from build123d import *

# Parameters (mm, degrees)
SKETCH1_W           = 44
SKETCH1_H           = 30
BOSS_EXTRUDE1_DEPTH = 3
SKETCH2_R           = 1
CUT_EXTRUDE1_DEPTH  = 5
SKETCH3_R           = 1
CUT_EXTRUDE2_DEPTH  = 5


with BuildPart() as part:
    # Sketch1 → Boss-Extrude1 (new body)
    with BuildSketch(Plane(origin=(0, 0, 0), x_dir=(1, 0, 0), z_dir=(0, 1, 0))):
        Rectangle(SKETCH1_W, SKETCH1_H)
    extrude(amount=BOSS_EXTRUDE1_DEPTH)

    # Sketch2 → Cut-Extrude1 (cut)
    with BuildSketch(Plane.ZY.offset(22)):
        with Locations((0, 1.5)):
            Circle(SKETCH2_R)
    cut_extrude1 = extrude(amount=-CUT_EXTRUDE1_DEPTH, mode=Mode.SUBTRACT)

    # Mirror1: Cut-Extrude1 across plane
    add(cut_extrude1.mirror(Plane(origin=(0, 0, 0), x_dir=(0, 0, 1), z_dir=(1, 0, 0))), mode=Mode.SUBTRACT)

    # Sketch3 → Cut-Extrude2 (cut)
    with BuildSketch(Plane(origin=(0, 0, 0), x_dir=(-1, 0, 0), z_dir=(0, -1, 0))):
        with Locations(Location((15, 4.5, 0), (0, 0, 90))):
            Circle(SKETCH3_R)
        with Locations(Location((15, -12.5, 0), (0, 0, 90))):
            Circle(SKETCH3_R)
        with Locations(Location((-15, -12.5, 0), (0, 0, 90))):
            Circle(SKETCH3_R)
        with Locations(Location((-15, 4.5, 0), (0, 0, 90))):
            Circle(SKETCH3_R)
    extrude(amount=-CUT_EXTRUDE2_DEPTH, mode=Mode.SUBTRACT)


solid = part.part
Read the model definition and answer for the solid it produces. Units are mm, in the model's axes. A direction names the side the tool comes from. Give positions to 0.01 mm unless a question says otherwise; leave off trailing zeros. Write each loop counter-clockwise with the first axis right and the second up, starting at its lowest first coordinate (ties: lowest second). Pieces come first, ordered by that corner, then holes. Notation, with made-up numbers: (62.25, -32.75) -> (88.25, -32.75) arc R15 ccw to (88.25, -8.75) -> close; hole circle Ø10 at (-34, 88.5). An arc over 180 degrees is marked (long way). Answer as a JSON object with one key per item and string values. Group by question number.
1) Find section C-C (y = 0.95). Write down the section's boundary in (x, z), and give its area (3 significant figures).
2) This flat-tipped pin is pushed along its axis until it touches: P1, Ø1.6, axis at y = 1.5, z = 0, coming from the +X side. Where does it stop, or does it pass through?
3) Find section B-B (x = 15). Write down the section's boundary in (y, z), and give its area (3 significant figures).
4) Find section A-A (z = 12.5). Write down the section's boundary in (x, y), and give its area (3 significant figures).
5) Consider L1, parallel to X at y = 1.2, z = 12.5; L2, parallel to Y at x = -21, z = 0; L3, parallel to X at y = 0.65, z = 13.25. Determine where each line is inside the solid, lowest interval first. Write a range as from..to.
6) A tool of negligible diameter and unlimited length cuts with its end or side. For faces 4 (the cylindrical face through (19.535, 0.524, -0.217)), 5 (the flat face through (22, 2.8, 0.2)), 6 (the cylindrical face through (-19.535, 0.524, -0.217)), from which of +Z, -Z, +X, -X, +Y, -Y can it reach the whole face along a straight path? Write none if from no direction.
7) The mould has two halves that part along X. Classify faces 1 (the flat face through (17, 2, 0)), 2 (the cylindrical face through (14.024, 1.479, -4.283)), 3 (the flat face through (0, 3, 0)): +X half, -X half, draft (parallel to the pull), parting line (faces both ways), or undercut.
8) Find section D-D (z = 0). Write down the section's boundary in (x, y), and give its area (3 significant figures).
Values follow:
{
 "1": {"outline": "(-22, -15) -> (22, -15) -> (22, -0.84) -> (17, -0.84) -> (17, 0.84) -> (22, 0.84) -> (22, 15) -> (-22, 15) -> (-22, 0.84) -> (-17, 0.84) -> (-17, -0.84) -> (-22, -0.84) -> close; hole circle Ø2 at (-15, -4.5); hole circle Ø2 at (-15, 12.5); hole circle Ø2 at (15, -4.5); hole circle Ø2 at (15, 12.5)", "area": "1,290 mm2"},
 "2": {"P1": "stops at x = 17"},
 "3": {"outline": "(0, -15) -> (3, -15) -> (3, -5.5) -> (0, -5.5) -> close; (0, -3.5) -> (3, -3.5) -> (3, 11.5) -> (0, 11.5) -> close; (0, 13.5) -> (3, 13.5) -> (3, 15) -> (0, 15) -> close", "area": "78.0 mm2"},
 "4": {"outline": "(-22, 0) -> (-16, 0) -> (-16, 3) -> (-22, 3) -> close; (-14, 0) -> (14, 0) -> (14, 3) -> (-14, 3) -> close; (16, 0) -> (22, 0) -> (22, 3) -> (16, 3) -> close", "area": "120 mm2"},
 "5": {"L1": "x = -22..-16, -14..14, 16..22", "L2": "y = 0..0.5, 2.5..3", "L3": "x = -22..-15.66, -14.34..14.34, 15.66..22"},
 "6": {"face 4": "+X", "face 5": "+Z, -Z, +X, +Y, -Y", "face 6": "-X"},
 "7": {"face 1": "+X half", "face 2": "undercut", "face 3": "draft"},
 "8": {"outline": "(-22, 0) -> (22, 0) -> (22, 0.5) -> (17, 0.5) -> (17, 2.5) -> (22, 2.5) -> (22, 3) -> (-22, 3) -> (-22, 2.5) -> (-17, 2.5) -> (-17, 0.5) -> (-22, 0.5) -> close", "area": "112 mm2"}
}
